from build123d import *

# Parameters (mm, degrees)
F1_DEPTH = 25


with BuildPart() as f1:
    # F0 (on Right) → F1 (new body)
    with BuildSketch(Plane.YZ):
        with BuildLine():
            Line((-42.287987, 69.438771), (-49.387987, 69.438771))
            Line((-49.387987, 69.438771), (-49.387987, -88.631229))
            Line((-49.387987, -88.631229), (-42.287987, -88.631229))
            Line((-42.287987, -88.631229), (-42.287987, 13.929646))
            Line((-42.287987, 13.929646), (-44.612987, 13.929646))
            ThreePointArc((-44.612987, 13.929646), (-46.734308, 14.808326), (-47.612987, 16.929646))
            Line((-47.612987, 16.929646), (-47.612987, 46.992207))
            ThreePointArc((-47.612987, 46.992207), (-46.734308, 49.113528), (-44.612987, 49.992207))
            Line((-44.612987, 49.992207), (-42.287987, 49.992207))
            Line((-42.287987, 49.992207), (-42.287987, 69.438771))
        make_face()
    extrude(amount=F1_DEPTH)


solid = f1.part
For this review, take the finished solid that the model builds, in its own axes (mm). A direction names the side the tool comes from. Round coordinates to 2 decimals unless told otherwise and drop trailing zeros. Order: outer loops, then holes, each group sorted by start corner. A loop starts at its lowest first (then second) coordinate and runs counter-clockwise, first axis right, second up. Notation, with made-up numbers: M 82,3 L 120,3 A16 ccw 120,22 Z; hole C 35.5,-2 d1. An arc over 180 degrees is marked long. Use a Markdown table: item, result. Add a question column.
Item 1: Add section C-C, the plane z = 37.5. Give the boundary of the cut face in (x, y).
Item 2: Mouldability with a two-part tool opening along Z and no side actions: class faces 3 (the flat face through (0, -46, -26)), 4 (the cylindrical face through (12.32, -46.76, 49.09)), 5 (the flat face through (12, -46, 69.439)) as released by +Z, released by -Z, zero draft, split by the parting line, or undercut.
Item 3: To check wall thickness, follow line 1 along Z through (x, y) = (23, -43); line 2 along Y through (x, z) = (11.5, 18.5); line 3 along Z through (x, y) = (14.5, -45). State the ranges of each line that lie inside material, in increasing order.
Item 4: Insertion check: pin 1 (7.5 mm diameter, centred on x = 11.5, z = 32.5, fed in from +Y). The pin has a flat end and moves straight along its axis. Give the tip position at first contact, or say it passes through.
Item 5: Add section B-B, the plane x = 5.5. Give the boundary of the cut face in (y, z).
Item 6: Tool access review of faces 1 (the flat face through (12, -46, -88.631)), 2 (the flat face through (12, -47.613, 32)): name each direction out of +Z, -Z, +X, -X, +Y, -Y from which nothing blocks a thin tool from reaching the whole face with its end or side.
Item 7: Add section A-A, the plane y = -43.5. Give the boundary of the cut face in (x, z), then the cut area to 3 significant figures.
Geometry results:
| question | item | result |
|---|---|---|
| 1 | outline | M 0,-49.39 L 25,-49.39 L 25,-47.61 L 0,-47.61 Z |
| 2 | face 3 | zero draft |
| 2 | face 4 | undercut |
| 2 | face 5 | released by +Z |
| 3 | line 1 | z = -88.63 to 13.93, 49.99 to 69.44 |
| 3 | line 2 | y = -49.39 to -47.61 |
| 3 | line 3 | z = -88.63 to 13.95, 49.97 to 69.44 |
| 4 | pin 1 | stops at y = -47.61 |
| 5 | outline | M -49.39,-88.63 L -42.29,-88.63 L -42.29,13.93 L -44.61,13.93 A3 cw -47.61,16.93 L -47.61,46.99 A3 cw -44.61,49.99 L -42.29,49.99 L -42.29,69.44 L -49.39,69.44 Z |
| 6 | face 1 | -Z, +X, -X, +Y, -Y |
| 6 | face 2 | +X, -X, +Y |
| 7 | outline | M 0,-88.63 L 25,-88.63 L 25,13.93 L 0,13.93 Z; M 0,49.99 L 25,49.99 L 25,69.44 L 0,69.44 Z |
| 7 | area | 3,050 mm² |
